For this review, take the finished solid that the model builds, in its own axes (mm). A direction names the side the tool comes from. Give positions to 0.01 mm unless a question says otherwise; leave off trailing zeros. Order: outer loops, then holes, each group sorted by start corner. A loop starts at its lowest first (then second) coordinate and runs counter-clockwise, first axis right, second up. Notation, with made-up numbers: (5.25, 75) - (33.25, 75) arc R24 ccw to (33.25, 113) - close; hole circle Ø4 at (8, 68.25). An arc over 180 degrees is marked (long way). One line per item, written item: value.
```python
from build123d import *

# Parameters (mm, degrees)
SKETCH2_R                = 3.81
BOSS_EXTRUDE1_DEPTH      = 2.54
SKETCH5_W                = 16.764
SKETCH5_H                = 6.35
BOSS_EXTRUDE2_DEPTH      = 16.51
SKETCH6_R                = 4.1275
CUT_EXTRUDE2_DEPTH       = 1.27
SKETCH7_R                = 1.27
CUT_EXTRUDE3_DEPTH       = 80.197102245
CUT_EXTRUDE4_DEPTH       = 2.286
BOSS_EXTRUDE3_DEPTH      = 3.81
F_4_CLEARANCE_HOLE1_D    = 2.9464
BOSS_EXTRUDE6_DEPTH      = 6.35
BOSS_EXTRUDE6_DEPTH_BACK = 2.54
SKETCH14_W               = 13.97
SKETCH14_H               = 3.81
FILLET1_R                = 5.08
CUT_EXTRUDE5_DEPTH       = 83.859689862
CUT_EXTRUDE5_DEPTH_BACK  = 83.859689862
SKETCH19_R               = 2.4892
BOSS_EXTRUDE8_DEPTH      = 2.54
CUT_EXTRUDE8_DEPTH       = 2.54
BOSS_EXTRUDE7_DEPTH      = 3.81
CUT_EXTRUDE7_DEPTH       = 87.868867767
SKETCH13_R               = 6.35
PRINT_TABS_DEPTH         = 0.4


# Read off the part's stored shape, not the designer's step: Boss-Extrude7
with BuildPart() as part:
    # Sketch2 → Boss-Extrude1 (new body)
    with BuildSketch(Plane.XY):
        with BuildLine():
            Line((-17.068825413, -8.459178389), (-41.402, 40.64))
            Line((-41.402, 40.64), (-41.402, 66.04))
            Line((-41.402, 66.04), (-1.524, 66.04))
            Line((-1.524, 66.04), (18.109053667, 5.913093546))
            ThreePointArc((18.109053667, 5.913093546), (7.204933647, -17.634949139), (-17.068825413, -8.459178389))
        make_face()
        Circle(SKETCH2_R, mode=Mode.SUBTRACT)
    extrude(amount=BOSS_EXTRUDE1_DEPTH)

    # Sketch5 → Boss-Extrude2 (add)
    with BuildSketch(Plane.XY.offset(2.54)):
        with Locations((-33.02, 43.815)):
            Rectangle(SKETCH5_W, SKETCH5_H)
    extrude(amount=BOSS_EXTRUDE2_DEPTH)

    # Sketch6 → Cut-Extrude2 (cut)
    with BuildSketch(Plane(origin=(0, 46.99, 0), x_dir=(1, 0, 0), z_dir=(0, 1, 0))):
        with Locations(Location((-33.02, -11.43, 0), (0, 0, 270))):
            Circle(SKETCH6_R)
    extrude(amount=-CUT_EXTRUDE2_DEPTH, mode=Mode.SUBTRACT)

    # Sketch7 → Cut-Extrude3 (cut, through all)
    with BuildSketch(Plane(origin=(0, 45.72, 0), x_dir=(1, 0, 0), z_dir=(0, 1, 0))):
        with Locations(Location((-33.02, -11.43, 0), (0, 0, 270))):
            Circle(SKETCH7_R)
    extrude(amount=-CUT_EXTRUDE3_DEPTH, mode=Mode.SUBTRACT)

    # Sketch9 → Cut-Extrude4 (cut)
    with BuildSketch(Plane(origin=(0, 0, 0), x_dir=(-1, 0, 0), z_dir=(0, 0, -1))):
        Polygon((3.171122265, 62.23), (5.077532854, 58.928), (8.890354032, 58.928), (10.796764621, 62.23), (8.890354032, 65.532), (5.077532854, 65.532), align=None)
        Polygon((24.379877895, 49.663956202), (23.308143816, 53.323053276), (19.603405755, 54.224452874), (16.970401774, 51.466755398), (18.042135853, 47.807658324), (21.746873914, 46.906258726), align=None)
        Polygon((5.918476139, 54.15579827), (4.846742059, 57.814895344), (1.142003999, 58.716294942), (-1.490999983, 55.958597466), (-0.419265903, 52.299500392), (3.285472157, 51.398100794), align=None)
    extrude(amount=-CUT_EXTRUDE4_DEPTH, mode=Mode.SUBTRACT)

    # Sketch8 → Boss-Extrude3 (add)
    with BuildSketch(Plane.XY.offset(2.54)):
        with BuildLine():
            Line((-15.367, 66.04), (-6.983943443, 66.04))
            Line((-6.983943443, 66.04), (-1.524, 66.04))
            Line((-1.524, 66.04), (3.09175139, 51.904101595))
            Line((3.09175139, 51.904101595), (-4.240438106, 50.120107003))
            Line((-4.240438106, 50.120107003), (-6.088713216, 57.716488409))
            Line((-6.088713216, 57.716488409), (-12.708473154, 56.10583501))
            ThreePointArc((-12.708473154, 56.10583501), (-14.673699407, 58.891843255), (-15.367, 62.23))
            Line((-15.367, 62.23), (-15.367, 66.04))
        make_face()
        Polygon((-17.142042414, 46.981018422), (-18.990317524, 54.577399829), (-26.415687706, 52.770733449), (-24.567412596, 45.174352043), align=None)
    extrude(amount=BOSS_EXTRUDE3_DEPTH)

    # #4 Clearance Hole1 (through all)
    with Locations(Plane.XY.offset(6.35)):
        with Locations((-6.983943443, 62.23), (-20.675139834, 50.5653558), (-2.213738078, 55.057197868)):
            Hole(F_4_CLEARANCE_HOLE1_D / 2)

    # Sketch14 → Boss-Extrude6 (add, two sides: drawn at the far end of the back side and taken through both)
    with BuildSketch(Plane.XY.offset(2.54).offset(-BOSS_EXTRUDE6_DEPTH_BACK)):
        with Locations((-13.968943443, 67.945)):
            Rectangle(SKETCH14_W, SKETCH14_H)
    extrude(amount=BOSS_EXTRUDE6_DEPTH + BOSS_EXTRUDE6_DEPTH_BACK)

    # Fillet1
    fillet1_edges = [part.edges().sort_by_distance(p)[0] for p in [
        (-41.402, 66.04, 1.27),
        (-1.524, 66.04, 3.175),
    ]]
    fillet(fillet1_edges, radius=FILLET1_R)

    # Sketch15 → Cut-Extrude5 (cut, two sides: drawn at the far end of the back side and taken through both)
    with BuildSketch(Plane.XY.offset(2.54).offset(-CUT_EXTRUDE5_DEPTH_BACK)):
        with BuildLine():
            ThreePointArc((-0.315167053, 48.411374113), (-18.310138041, 44.816284079), (-33.674369734, 34.782140486))
            ThreePointArc((-33.674369734, 34.782140486), (-33.731327517, 31.262340905), (-30.211527936, 31.205383122))
            ThreePointArc((-30.211527936, 31.205383122), (-16.427248714, 40.207684038), (-0.28275743, 43.433079608))
            ThreePointArc((-0.28275743, 43.433079608), (2.190185011, 45.938431672), (-0.315167053, 48.411374113))
        make_face()
    extrude(amount=CUT_EXTRUDE5_DEPTH + CUT_EXTRUDE5_DEPTH_BACK, mode=Mode.SUBTRACT)

    # Sketch19 → Boss-Extrude8 (add, through all)
    with BuildSketch(Plane.XY.offset(2.54)):
        with BuildLine():
            Line((5.466200245, 44.632269783), (-40.158007355, -3.769954845))
            ThreePointArc((-40.158007355, -3.769954845), (-46.15516131, -4.814733016), (-48.848797168, 0.64436424))
            Line((-48.848797168, 0.64436424), (-41.402, 40.64))
            Line((-41.402, 40.64), (3.09175139, 51.904101595))
            Line((3.09175139, 51.904101595), (5.466200245, 44.632269783))
        make_face()
        with Locations((-0.298962241, 45.92222686)):
            Circle(SKETCH19_R, mode=Mode.SUBTRACT)
        with Locations((-43.854625645, -0.285501773)):
            Circle(SKETCH19_R, mode=Mode.SUBTRACT)
    extrude(amount=-BOSS_EXTRUDE8_DEPTH)

    # Sketch20 → Cut-Extrude8 (cut)
    with BuildSketch(Plane.XY.offset(2.54)):
        Polygon((-40.158007355, -3.769954845), (10.729493517, 49.863783044), (48.07174347, 14.433588323), (-7.673080914, -44.319607422), align=None)
    extrude(amount=-CUT_EXTRUDE8_DEPTH, mode=Mode.SUBTRACT)

    # Boss-Extrude7 outline → Boss-Extrude7 (add)
    with BuildSketch(Plane.XY.offset(2.54)):
        with BuildLine():
            ThreePointArc((-19.720952416, 49.442927803), (-20.146011494, 49.271262362), (-20.56957647, 49.095942783))
            ThreePointArc((-20.56957647, 49.095942783), (-20.117584831, 49.201739043), (-19.720952416, 49.442927803))
        make_face()
        with BuildLine():
            ThreePointArc((-24.638, 43.697782335), (-21.550057665, 45.300355844), (-18.358466971, 46.685050235))
            Line((-18.358466971, 46.685050235), (-24.567412596, 45.174352043))
            Line((-24.567412596, 45.174352043), (-24.638, 45.464465155))
            Line((-24.638, 45.464465155), (-24.638, 43.697782335))
        make_face()
        with BuildLine():
            ThreePointArc((-4.941378488, 53.000960864), (-11.514519488, 51.97051967), (-17.907769463, 50.128144457))
            Line((-17.907769463, 50.128144457), (-17.178757335, 47.131916166))
            ThreePointArc((-17.178757335, 47.131916166), (-6.891074176, 49.689438734), (3.704334892, 50.028043416))
            Line((3.704334892, 50.028043416), (3.09175139, 51.904101595))
            Line((3.09175139, 51.904101595), (-4.240438106, 50.120107003))
            Line((-4.240438106, 50.120107003), (-4.941378488, 53.000960864))
        make_face()
    extrude(amount=BOSS_EXTRUDE7_DEPTH)

    # Sketch16 → Cut-Extrude7 (cut, through all)
    with BuildSketch(Plane.XY.offset(2.54)):
        with BuildLine():
            ThreePointArc((-0.326576563, 50.163936974), (-18.972991936, 46.4386994), (-34.893431388, 36.041305068))
            ThreePointArc((-34.893431388, 36.041305068), (-34.990492099, 30.043279251), (-28.992466282, 29.94621854))
            ThreePointArc((-28.992466282, 29.94621854), (-15.764394819, 38.585268717), (-0.271347919, 41.680516747))
            ThreePointArc((-0.271347919, 41.680516747), (3.942747872, 45.949841182), (-0.326576563, 50.163936974))
        make_face()
    extrude(amount=CUT_EXTRUDE7_DEPTH, mode=Mode.SUBTRACT)

    # Sketch13 → Print Tabs (add)
    with BuildSketch(Plane(origin=(0, 0, 0), x_dir=(-1, 0, 0), z_dir=(0, 0, -1))):
        with Locations((14.284313144, 23.500060577)):
            Circle(SKETCH13_R)
        with Locations((21.463, 66.04)):
            Circle(SKETCH13_R)
        with Locations((41.402, 40.64)):
            Circle(SKETCH13_R)
    extrude(amount=-PRINT_TABS_DEPTH)


solid = part.part
```
(1) Take a section at C-C (y = 7). Write out the cut boundary in (x, z), then the cut area to 3 significant figures.
Answers below:
outline: (-47.67, 0) - (-30.01, 0) - (-30.01, 2.54) - (-47.67, 2.54) - close
area: 44.9 mm^2
(2) For P1, Ø10, axis at y = 54, z = 6.5, coming from the -X side; P2, Ø8.5, axis at x = -11.5, y = 23, coming from the +Z side; P3, Ø6, axis at x = -37, z = 13, coming from the -Y side; P4, Ø2, axis at x = -42, y = 19.5, coming from the -Z side, all flat-tipped, find the tip position at first contact; note any pin that passes through.
Answers below:
P1: stops at x = -41.4
P2: stops at z = 2.54
P3: stops at y = 40.64
P4: stops at z = 0
(3) Draft analysis for pull direction Y (two halves, no side actions). For faces 5 (the face through (-33.26, 3.55, 1.29)), 6 (the face through (-3.02, 58.26, 1.13)), 7 (the face through (-14, 69.85, 4)), state which applies: pulls with the +Y half, pulls with the -Y half, needs draft (parallel to the pull), parting line crosses it, or undercut.
Answers below:
face 5: pulls with the -Y half
face 6: undercut
face 7: pulls with the +Y half
(4) Take a section at D-D (y = 23). Write out the cut boundary in (x, z).
Answers below:
outline: (-44.69, 0) - (-7.95, 0) - (-7.95, 0.4) - (-14.76, 0.4) - (-14.76, 2.54) - (-44.69, 2.54) - close
(5) Take a section at A-A (x = -33.02). Write out the cut boundary in (y, z).
Answers below:
outline: (3.8, 0) - (66.04, 0) - (66.04, 2.54) - (46.99, 2.54) - (46.99, 7.3) - (45.72, 7.3) - (45.72, 10.16) - (40.64, 10.16) - (40.64, 2.54) - (3.8, 2.54) - close; (40.64, 12.7) - (45.72, 12.7) - (45.72, 15.56) - (46.99, 15.56) - (46.99, 19.05) - (40.64, 19.05) - close
(6) Take a section at B-B (x = -44.5). Write out the cut boundary in (y, z), then the cut area to 3 significant figures.
Answers below:
outline: (-5.32, 0) - (-2.69, 0) - (-2.69, 2.54) - (-5.32, 2.54) - close; (2.12, 0) - (24, 0) - (24, 2.54) - (2.12, 2.54) - close; (35.1, 0) - (46.18, 0) - (46.18, 0.4) - (35.1, 0.4) - close
area: 66.7 mm^2
(7) Wall thickness on line 1 (Z direction, x = -38, y = 55); line 2 (Y direction, x = -10, z = 3); line 3 (X direction, y = 46.7, z = 11.43): over which ranges is each line inside the solid? List them lowest first. Write a range as from..to.
Answers below:
line 1: z = 0..2.54
line 2: y = 49.16..52.28, 56.76..69.85
line 3: x = -41.4..-37.15, -28.89..-24.64
(8) Machinability: for faces 1 (the face through (-27, 57, 2.54)), 2 (the face through (-25.722, 49.921, 4.418)), 3 (the face through (-1.407, 51.855, 1.127)), 4 (the face through (-41.402, 46, 7)), which of the approach directions +Z, -Z, +X, -X, +Y, -Y give a long, thin tool a straight path to every point of the face, cutting with its end or side? Answer none if there is none.
Answers below:
face 1: +Z
face 2: +Z, -X
face 3: -Z
face 4: +Z, -X, +Y
